Work out the finished part from the listing and answer in its coordinate system (mm). A direction names the side the tool comes from. Round coordinates to 2 decimals unless told otherwise and drop trailing zeros. Write each loop counter-clockwise with the first axis right and the second up, starting at its lowest first coordinate (ties: lowest second). Pieces come first, ordered by that corner, then holes. Notation, with made-up numbers: (6.25, 66.25) - (36.25, 66.25) arc R20 cw to (36.25, 89.25) - close; hole circle Ø2 at (-13.5, -19.5). An arc over 180 degrees is marked (long way). Write item = value, one per line. Start each with the question number.
from build123d import *

# Parameters (mm, degrees)
F1_DEPTH = 10
F2_DEPTH = 4
F3_D     = 6.6
F4_R     = 6
F4_R_2   = 3.3
F5_DEPTH = 4


with BuildPart() as f1:
    # F0 (on Top) → F1 (new body)
    with BuildSketch(Plane.XY):
        with BuildLine():
            Line((5.930585, 22.739353), (16.505714, 16.727564))
            ThreePointArc((16.505714, 16.727564), (11.613883, 20.42958), (5.930585, 22.739353))
        make_face()
        with BuildLine():
            Line((-22.65815, -6.233639), (-22.739353, 5.930585))
            ThreePointArc((-22.739353, 5.930585), (-23.499476, -0.156872), (-22.65815, -6.233639))
        make_face()
        with BuildLine():
            ThreePointArc((6.233639, -22.65815), (11.885593, -20.272708), (16.727564, -16.505714))
            Line((16.727564, -16.505714), (6.233639, -22.65815))
        make_face()
        with BuildLine():
            ThreePointArc((16.727564, -16.505714), (11.964046, 0.079867), (16.505714, 16.727564))
            Line((16.505714, 16.727564), (5.930585, 22.739353))
            ThreePointArc((5.930585, 22.739353), (-6.05119, 10.321235), (-22.739353, 5.930585))
            Line((-22.739353, 5.930585), (-22.65815, -6.233639))
            ThreePointArc((-22.65815, -6.233639), (-5.912857, -10.401101), (6.233639, -22.65815))
            Line((6.233639, -22.65815), (16.727564, -16.505714))
        make_face()
        Polygon((-5.15, 2.973354), (0, 5.946708), (5.15, 2.973354), (5.15, -2.973354), (0, -5.946708), (-5.15, -2.973354), align=None, mode=Mode.SUBTRACT)
        Polygon((5.15, 2.973354), (0, 5.946708), (-5.15, 2.973354), (-5.15, -2.973354), (0, -5.946708), (5.15, -2.973354), align=None)
    extrude(amount=F1_DEPTH)

    # F0 (on Top) → F2 (cut)
    with BuildSketch(Plane.XY):
        Polygon((5.15, 2.973354), (0, 5.946708), (-5.15, 2.973354), (-5.15, -2.973354), (0, -5.946708), (5.15, -2.973354), align=None)
    extrude(amount=F2_DEPTH, mode=Mode.SUBTRACT)

    # F3 (through all)
    with Locations(Plane(origin=(0, 0, 0), x_dir=(1, 0, 0), z_dir=(0, 0, -1))):
        with Locations((0, 0)):
            Hole(F3_D / 2)

    # F4 (on face) → F5 (cut)
    with BuildSketch(Plane.XY.offset(10)):
        Circle(F4_R)
        Circle(F4_R_2, mode=Mode.SUBTRACT)
    extrude(amount=-F5_DEPTH, mode=Mode.SUBTRACT)


solid = f1.part
1. Which of the six approach directions +Z, -Z, +X, -X, +Y, -Y give full straight-line access (tool end or side, diameter ignored) to faces 1 (the face through (-6, 0, 8)), 2 (the face through (-2, -3, 4)), 3 (the face through (11.689, 20.387, 4.93))?
2. Consider line 1 (Y direction, x = 0, z = 4.5); line 2 (Y direction, x = -1, z = 5.75); line 3 (Z direction, x = -3, y = 4.5). Determine where each line is inside the solid, lowest interval first.
3. Find section B-B on y = 0. Give the vertices of the cut face in (x, z).
4. Each of these flat-tipped pins is pushed along its axis until it touches: pin 1 (3 mm diameter, centred on y = -2.5, z = 8.5, fed in from +X); pin 2 (6 mm diameter, centred on x = 3, z = 1.5, fed in from -Y); pin 3 (2 mm diameter, centred on y = -0.5, z = 1.5, fed in from +X). Where does it stop, or does it pass through?
5. Find section C-C on z = 1.75. Give the vertices of the cut face in (x, y).
6. Find section D-D on x = -12.5. Give the vertices of the cut face in (y, z).
7. Find section A-A on z = 7.25. Give the vertices of the cut face in (x, y).
8. For a pull along Y with two mould halves and no side action, classify faces 4 (the face through (11.811, -20.316, 4.93)), 5 (the face through (-23.5, -0.1, 4.9)), 6 (the face through (2.61, 4.44, 1.97)) as released by +Y, released by -Y, zero draft, split by the parting line, or undercut.
Answer key:
q1.face_1 = +Z
q1.face_2 = -Z
q1.face_3 = +Z, -Z, +X, +Y
q2.line_1 = -14.73 to -3.3, 3.3 to 14.91
q2.line_2 = -13.84 to -3.14, 3.14 to 13.99
q2.line_3 = 0 to 6
q3.outline = (-23.5, 0) - (-5.15, 0) - (-5.15, 4) - (-3.3, 4) - (-3.3, 6) - (-6, 6) - (-6, 10) - (-23.5, 10) - close; (3.3, 4) - (5.15, 4) - (5.15, 0) - (11.96, 0) - (11.96, 10) - (6, 10) - (6, 6) - (3.3, 6) - close
q4.pin_1 = 12.25
q4.pin_2 = -22.25
q4.pin_3 = 12.01
q5.outline = (-22.74, 5.93) arc R23.5 ccw to (-22.66, -6.23) arc R32 cw to (6.23, -22.66) arc R23.5 ccw to (16.73, -16.51) arc R32 cw to (16.51, 16.73) arc R23.5 ccw to (5.93, 22.74) arc R32 cw to start; hole (-5.15, -2.97) - (0, -5.95) - (5.15, -2.97) - (5.15, 2.97) - (0, 5.95) - (-5.15, 2.97) - close
q6.outline = (-7.58, 0) - (7.44, 0) - (7.44, 10) - (-7.58, 10) - close
q7.outline = (-22.74, 5.93) arc R23.5 ccw to (-22.66, -6.23) arc R32 cw to (6.23, -22.66) arc R23.5 ccw to (16.73, -16.51) arc R32 cw to (16.51, 16.73) arc R23.5 ccw to (5.93, 22.74) arc R32 cw to start; hole circle Ø12 at (0, 0)
q8.face_4 = released by -Y
q8.face_5 = split by the parting line
q8.face_6 = undercut
